Part model, mm, in its own coordinate system. A direction names the side the tool comes from. Give positions to 0.01 mm unless a question says otherwise; leave off trailing zeros. Order: outer loops, then holes, each group sorted by start corner. A loop starts at its lowest first (then second) coordinate and runs counter-clockwise, first axis right, second up.
1. Mould opens along Z. For faces 1 (the flat face through (0, 0, 1)), 2 (the flat face through (7, 7, 0)), 3 (the flat face through (6.8, -6.2, 11)) say: +Z half, -Z half, draft (parallel to the pull), parting line (faces both ways), or undercut.
2. Which spindle directions (+Z, -Z, +X, -X, +Y, -Y) get a long thin tool onto all of the face, cutting with end or side? Do faces 4 (the flat face through (-5.5, -0.1, 12)), 5 (the flat face through (-1.2, 5, 5.9)), 6 (the flat face through (-7, 5.5, 6.1)). Say none if no direction does.
3. Slice it at C-C on y = -4.25. List the corners of the cut face in (x, z), and give its area (3 significant figures).
4. Slice it at B-B on x = 6.5. List the corners of the cut face in (y, z).
5. Slice it at A-A on z = 6. Give the number of separate pieces and of enclosed holes in the cut face, and give its area (3 significant figures).
6. Probe line 1 (X direction, y = -4.5, z = 0.25); line 2 (X direction, y = -1.05, z = 6); line 3 (Y direction, x = -1.5, z = 6). List the from-to ranges inside material, lowest first.
7. Slice it at D-D on x = 3.5. List the corners of the cut face in (y, z).
8. Drop flat-ended pins along their axis: pin 1 Ø0.6 at (x, z) = (6.5, 4.5) entering from +Y; pin 2 Ø2.5 at (y, z) = (0, 6) entering from +X; pin 3 Ø6 at (y, z) = (0, 1) entering from -X. Give the stop position or say it passes through.
from build123d import *

# Parameters (mm, degrees)
SKETCH1_W            = 12
SKETCH1_H            = 12
BOSS_EXTRUDE1_DEPTH  = 12
SKETCH2_W            = 10
SKETCH2_H            = 12
CUT_EXTRUDE1_DEPTH   = 1
SKETCH3_W            = 10
SKETCH3_H            = 11
CUT_EXTRUDE2_DEPTH   = 1
SKETCH4_W            = 10
SKETCH4_H            = 11
CUT_EXTRUDE3_DEPTH   = 1
SKETCH5_W            = 10
SKETCH5_H            = 10
CUT_EXTRUDE4_DEPTH   = 1
SKETCH6_W            = 12
SKETCH6_H            = 1
BOSS_EXTRUDE2_DEPTH  = 1
SKETCH7_W            = 12
SKETCH7_H            = 1
BOSS_EXTRUDE3_DEPTH  = 1
SKETCH8_W            = 12
SKETCH8_H            = 1
BOSS_EXTRUDE4_DEPTH  = 1
SKETCH12_W           = 2
SKETCH12_H           = 1
BOSS_EXTRUDE5_DEPTH  = 1
SKETCH13_W           = 2
SKETCH13_H           = 1
BOSS_EXTRUDE6_DEPTH  = 1
SKETCH14_W           = 2
SKETCH14_H           = 1
BOSS_EXTRUDE7_DEPTH  = 1
SKETCH16_W           = 2
SKETCH16_H           = 1
BOSS_EXTRUDE8_DEPTH  = 1
SKETCH19_W           = 2
SKETCH19_H           = 1
BOSS_EXTRUDE10_DEPTH = 1
SKETCH20_W           = 2
SKETCH20_H           = 1
BOSS_EXTRUDE11_DEPTH = 1
SKETCH21_W           = 2
SKETCH21_H           = 1
BOSS_EXTRUDE12_DEPTH = 1
SKETCH22_W           = 2
SKETCH22_H           = 1
BOSS_EXTRUDE13_DEPTH = 1
SKETCH23_W           = 1
SKETCH23_H           = 2
BOSS_EXTRUDE15_DEPTH = 1
SKETCH24_W           = 3
SKETCH24_H           = 2
BOSS_EXTRUDE16_DEPTH = 1
SKETCH25_W           = 1
SKETCH25_H           = 2
BOSS_EXTRUDE17_DEPTH = 1
SKETCH26_W           = 1
SKETCH26_H           = 2
BOSS_EXTRUDE19_DEPTH = 1
SKETCH28_W           = 1
SKETCH28_H           = 2
BOSS_EXTRUDE20_DEPTH = 1
SKETCH29_W           = 1
SKETCH29_H           = 2
BOSS_EXTRUDE21_DEPTH = 1
SKETCH30_W           = 1
SKETCH30_H           = 2
BOSS_EXTRUDE22_DEPTH = 1
SKETCH31_W           = 1
SKETCH31_H           = 2
BOSS_EXTRUDE24_DEPTH = 1
SKETCH33_W           = 1
SKETCH33_H           = 2
BOSS_EXTRUDE25_DEPTH = 1
SKETCH34_W           = 3
SKETCH34_H           = 2
BOSS_EXTRUDE26_DEPTH = 1
SKETCH35_W           = 3
SKETCH35_H           = 2
BOSS_EXTRUDE27_DEPTH = 1
SKETCH36_W           = 3
SKETCH36_H           = 2
BOSS_EXTRUDE28_DEPTH = 1
SKETCH37_W           = 3
SKETCH37_H           = 2
BOSS_EXTRUDE29_DEPTH = 1
SKETCH38_W           = 3
SKETCH38_H           = 2
BOSS_EXTRUDE30_DEPTH = 1
SKETCH39_W           = 3
SKETCH39_H           = 2
BOSS_EXTRUDE31_DEPTH = 1
SKETCH40_W           = 3
SKETCH40_H           = 2
BOSS_EXTRUDE32_DEPTH = 1
SKETCH41_R           = 1
CUT_EXTRUDE6_DEPTH   = 12
SKETCH42_R           = 1
CUT_EXTRUDE7_DEPTH   = 12


with BuildPart() as part:
    # Sketch1 → Boss-Extrude1 (new body)
    with BuildSketch(Plane.XY):
        Rectangle(SKETCH1_W, SKETCH1_H)
    extrude(amount=BOSS_EXTRUDE1_DEPTH)

    # Sketch2 → Cut-Extrude1 (cut)
    with BuildSketch(Plane.XY.offset(12)):
        Rectangle(SKETCH2_W, SKETCH2_H)
    extrude(amount=-CUT_EXTRUDE1_DEPTH, mode=Mode.SUBTRACT)

    # Sketch3 → Cut-Extrude2 (cut)
    with BuildSketch(Plane(origin=(0, -6, 0), x_dir=(-1, 0, 0), z_dir=(0, -1, 0))):
        with Locations((0, -5.5)):
            Rectangle(SKETCH3_W, SKETCH3_H)
    extrude(amount=-CUT_EXTRUDE2_DEPTH, mode=Mode.SUBTRACT)

    # Sketch4 → Cut-Extrude3 (cut)
    with BuildSketch(Plane(origin=(0, 0, 0), x_dir=(-1, 0, 0), z_dir=(0, 0, -1))):
        with Locations((0, 0.5)):
            Rectangle(SKETCH4_W, SKETCH4_H)
    extrude(amount=-CUT_EXTRUDE3_DEPTH, mode=Mode.SUBTRACT)

    # Sketch5 → Cut-Extrude4 (cut)
    with BuildSketch(Plane(origin=(0, 6, 0), x_dir=(1, 0, 0), z_dir=(0, 1, 0))):
        with Locations((0, -6)):
            Rectangle(SKETCH5_W, SKETCH5_H)
    extrude(amount=-CUT_EXTRUDE4_DEPTH, mode=Mode.SUBTRACT)

    # Sketch6 → Boss-Extrude2 (add)
    with BuildSketch(Plane.ZY.offset(6)):
        with Locations((6, -5.5)):
            Rectangle(SKETCH6_W, SKETCH6_H)
    extrude(amount=BOSS_EXTRUDE2_DEPTH)

    # Sketch7 → Boss-Extrude3 (add)
    with BuildSketch(Plane.ZY.offset(6)):
        with Locations((6, 5.5)):
            Rectangle(SKETCH7_W, SKETCH7_H)
    extrude(amount=BOSS_EXTRUDE3_DEPTH)

    # Sketch8 → Boss-Extrude4 (add)
    with BuildSketch(Plane(origin=(6, 0, 0), x_dir=(0, 0, -1), z_dir=(1, 0, 0))):
        with Locations((-6, 5.5)):
            Rectangle(SKETCH8_W, SKETCH8_H)
        with Locations((-6, -5.5)):
            Rectangle(SKETCH8_W, SKETCH8_H)
    extrude(amount=BOSS_EXTRUDE4_DEPTH)

    # Sketch12 → Boss-Extrude5 (add)
    with BuildSketch(Plane(origin=(0, -6, 0), x_dir=(-1, 0, 0), z_dir=(0, -1, 0))):
        with Locations((-6, -0.5)):
            Rectangle(SKETCH12_W, SKETCH12_H)
    extrude(amount=BOSS_EXTRUDE5_DEPTH)

    # Sketch13 → Boss-Extrude6 (add)
    with BuildSketch(Plane(origin=(0, -6, 0), x_dir=(-1, 0, 0), z_dir=(0, -1, 0))):
        with Locations((-6, -11.5)):
            Rectangle(SKETCH13_W, SKETCH13_H)
    extrude(amount=BOSS_EXTRUDE6_DEPTH)

    # Sketch14 → Boss-Extrude7 (add)
    with BuildSketch(Plane(origin=(0, -6, 0), x_dir=(-1, 0, 0), z_dir=(0, -1, 0))):
        with Locations((6, -0.5)):
            Rectangle(SKETCH14_W, SKETCH14_H)
    extrude(amount=BOSS_EXTRUDE7_DEPTH)

    # Sketch16 → Boss-Extrude8 (add)
    with BuildSketch(Plane(origin=(0, -6, 0), x_dir=(-1, 0, 0), z_dir=(0, -1, 0))):
        with Locations((6, -11.5)):
            Rectangle(SKETCH16_W, SKETCH16_H)
    extrude(amount=BOSS_EXTRUDE8_DEPTH)

    # Sketch19 → Boss-Extrude10 (add)
    with BuildSketch(Plane(origin=(0, 6, 0), x_dir=(1, 0, 0), z_dir=(0, 1, 0))):
        with Locations((6, -11.5)):
            Rectangle(SKETCH19_W, SKETCH19_H)
    extrude(amount=BOSS_EXTRUDE10_DEPTH)

    # Sketch20 → Boss-Extrude11 (add)
    with BuildSketch(Plane(origin=(0, 6, 0), x_dir=(1, 0, 0), z_dir=(0, 1, 0))):
        with Locations((-6, -11.5)):
            Rectangle(SKETCH20_W, SKETCH20_H)
    extrude(amount=BOSS_EXTRUDE11_DEPTH)

    # Sketch21 → Boss-Extrude12 (add)
    with BuildSketch(Plane(origin=(0, 6, 0), x_dir=(1, 0, 0), z_dir=(0, 1, 0))):
        with Locations((6, -0.5)):
            Rectangle(SKETCH21_W, SKETCH21_H)
    extrude(amount=BOSS_EXTRUDE12_DEPTH)

    # Sketch22 → Boss-Extrude13 (add)
    with BuildSketch(Plane(origin=(0, 6, 0), x_dir=(1, 0, 0), z_dir=(0, 1, 0))):
        with Locations((-6, -0.5)):
            Rectangle(SKETCH22_W, SKETCH22_H)
    extrude(amount=BOSS_EXTRUDE13_DEPTH)

    # Sketch23 → Boss-Extrude15 (add)
    with BuildSketch(Plane(origin=(7, 0, 0), x_dir=(0, 0, -1), z_dir=(1, 0, 0))):
        with Locations((-11.5, 6)):
            Rectangle(SKETCH23_W, SKETCH23_H)
    extrude(amount=BOSS_EXTRUDE15_DEPTH)

    # Sketch24 → Boss-Extrude16 (add)
    with BuildSketch(Plane.XY.offset(12)):
        with Locations((6.5, 6)):
            Rectangle(SKETCH24_W, SKETCH24_H)
    extrude(amount=BOSS_EXTRUDE16_DEPTH)

    # Sketch25 → Boss-Extrude17 (add)
    with BuildSketch(Plane(origin=(7, 0, 0), x_dir=(0, 0, -1), z_dir=(1, 0, 0))):
        with Locations((-11.5, -6)):
            Rectangle(SKETCH25_W, SKETCH25_H)
    extrude(amount=BOSS_EXTRUDE17_DEPTH)

    # Sketch26 → Boss-Extrude19 (add)
    with BuildSketch(Plane(origin=(7, 0, 0), x_dir=(0, 0, -1), z_dir=(1, 0, 0))):
        with Locations((-0.5, -6)):
            Rectangle(SKETCH26_W, SKETCH26_H)
    extrude(amount=BOSS_EXTRUDE19_DEPTH)

    # Sketch28 → Boss-Extrude20 (add)
    with BuildSketch(Plane(origin=(7, 0, 0), x_dir=(0, 0, -1), z_dir=(1, 0, 0))):
        with Locations((-0.5, 6)):
            Rectangle(SKETCH28_W, SKETCH28_H)
    extrude(amount=BOSS_EXTRUDE20_DEPTH)

    # Sketch29 → Boss-Extrude21 (add)
    with BuildSketch(Plane.ZY.offset(7)):
        with Locations((0.5, 6)):
            Rectangle(SKETCH29_W, SKETCH29_H)
    extrude(amount=BOSS_EXTRUDE21_DEPTH)

    # Sketch30 → Boss-Extrude22 (add)
    with BuildSketch(Plane.ZY.offset(7)):
        with Locations((11.5, 6)):
            Rectangle(SKETCH30_W, SKETCH30_H)
    extrude(amount=BOSS_EXTRUDE22_DEPTH)

    # Sketch31 → Boss-Extrude24 (add)
    with BuildSketch(Plane.ZY.offset(7)):
        with Locations((0.5, -6)):
            Rectangle(SKETCH31_W, SKETCH31_H)
    extrude(amount=BOSS_EXTRUDE24_DEPTH)

    # Sketch33 → Boss-Extrude25 (add)
    with BuildSketch(Plane.ZY.offset(7)):
        with Locations((11.5, -6)):
            Rectangle(SKETCH33_W, SKETCH33_H)
    extrude(amount=BOSS_EXTRUDE25_DEPTH)

    # Sketch34 → Boss-Extrude26 (add)
    with BuildSketch(Plane.XY.offset(12)):
        with Locations((-6.5, 6)):
            Rectangle(SKETCH34_W, SKETCH34_H)
    extrude(amount=BOSS_EXTRUDE26_DEPTH)

    # Sketch35 → Boss-Extrude27 (add)
    with BuildSketch(Plane.XY.offset(12)):
        with Locations((-6.5, -6)):
            Rectangle(SKETCH35_W, SKETCH35_H)
    extrude(amount=BOSS_EXTRUDE27_DEPTH)

    # Sketch36 → Boss-Extrude28 (add)
    with BuildSketch(Plane.XY.offset(12)):
        with Locations((6.5, -6)):
            Rectangle(SKETCH36_W, SKETCH36_H)
    extrude(amount=BOSS_EXTRUDE28_DEPTH)

    # Sketch37 → Boss-Extrude29 (add)
    with BuildSketch(Plane(origin=(0, 0, 0), x_dir=(-1, 0, 0), z_dir=(0, 0, -1))):
        with Locations((-6.5, 6)):
            Rectangle(SKETCH37_W, SKETCH37_H)
    extrude(amount=BOSS_EXTRUDE29_DEPTH)

    # Sketch38 → Boss-Extrude30 (add)
    with BuildSketch(Plane(origin=(0, 0, 0), x_dir=(-1, 0, 0), z_dir=(0, 0, -1))):
        with Locations((-6.5, -6)):
            Rectangle(SKETCH38_W, SKETCH38_H)
    extrude(amount=BOSS_EXTRUDE30_DEPTH)

    # Sketch39 → Boss-Extrude31 (add)
    with BuildSketch(Plane(origin=(0, 0, 0), x_dir=(-1, 0, 0), z_dir=(0, 0, -1))):
        with Locations((6.5, -6)):
            Rectangle(SKETCH39_W, SKETCH39_H)
    extrude(amount=BOSS_EXTRUDE31_DEPTH)

    # Sketch40 → Boss-Extrude32 (add)
    with BuildSketch(Plane(origin=(0, 0, 0), x_dir=(-1, 0, 0), z_dir=(0, 0, -1))):
        with Locations((6.5, 6)):
            Rectangle(SKETCH40_W, SKETCH40_H)
    extrude(amount=BOSS_EXTRUDE32_DEPTH)

    # Sketch41 → Cut-Extrude6 (cut)
    with BuildSketch(Plane(origin=(6, 0, 0), x_dir=(0, 0, -1), z_dir=(1, 0, 0))):
        with Locations((-6, 0)):
            Circle(SKETCH41_R)
    extrude(amount=-CUT_EXTRUDE6_DEPTH, mode=Mode.SUBTRACT)

    # Sketch42 → Cut-Extrude7 (cut)
    with BuildSketch(Plane(origin=(0, -5, 0), x_dir=(-1, 0, 0), z_dir=(0, -1, 0))):
        with Locations(Location((0, -6, 0), (0, 0, 90))):
            Circle(SKETCH42_R)
    extrude(amount=-CUT_EXTRUDE7_DEPTH, mode=Mode.SUBTRACT)


solid = part.part
Data:
1. face 1: -Z half
1. face 2: draft
1. face 3: undercut
2. face 4: +Z, +X, -X
2. face 5: +Z, -Z, +Y
2. face 6: -X, +Y, -Y
3. outline: (-6, 0) - (-5, 0) - (-5, 1) - (5, 1) - (5, 0) - (6, 0) - (6, 12) - (5, 12) - (5, 11) - (-5, 11) - (-5, 12) - (-6, 12) - close; hole circle Ø2 at (0, 6)
3. area: 121 mm2
4. outline: (-7, -1) - (-5, -1) - (-5, 13) - (-7, 13) - (-7, 11) - (-6, 11) - (-6, 1) - (-7, 1) - close; (5, -1) - (7, -1) - (7, 1) - (6, 1) - (6, 11) - (7, 11) - (7, 13) - (5, 13) - close
5. separate pieces: 4
5. enclosed holes: 0
5. area: 88.0 mm2
6. line 1: x = -6 to -5, 5 to 6
6. line 2: x = -6 to -1, 1 to 6
6. line 3: y = -5 to -1, 1 to 5
7. outline: (-5, 1) - (5, 1) - (5, 11) - (-5, 11) - close; hole circle Ø2 at (0, 6)
8. pin 1: stops at y = 6
8. pin 2: stops at x = 6
8. pin 3: stops at x = -6
